Design review of the part shown in the three views and the two pictorial views. Dimensions are in mm from the part's minimum x, y and z. A direction names the side the tool comes from. Give positions to 0.01 mm unless a question says otherwise; leave off trailing zeros. Order: outer loops, then holes, each group sorted by start corner. A loop starts at its lowest first (then second) coordinate and runs counter-clockwise, first axis right, second up. Notation, with made-up numbers: (17.5, 66.5) -> (42.5, 66.5) arc R21 ccw to (42.5, 85.5) -> close; hole circle Ø5 at (51.5, 65.5). An arc over 180 degrees is marked (long way). Use one line per item in the form item = value.
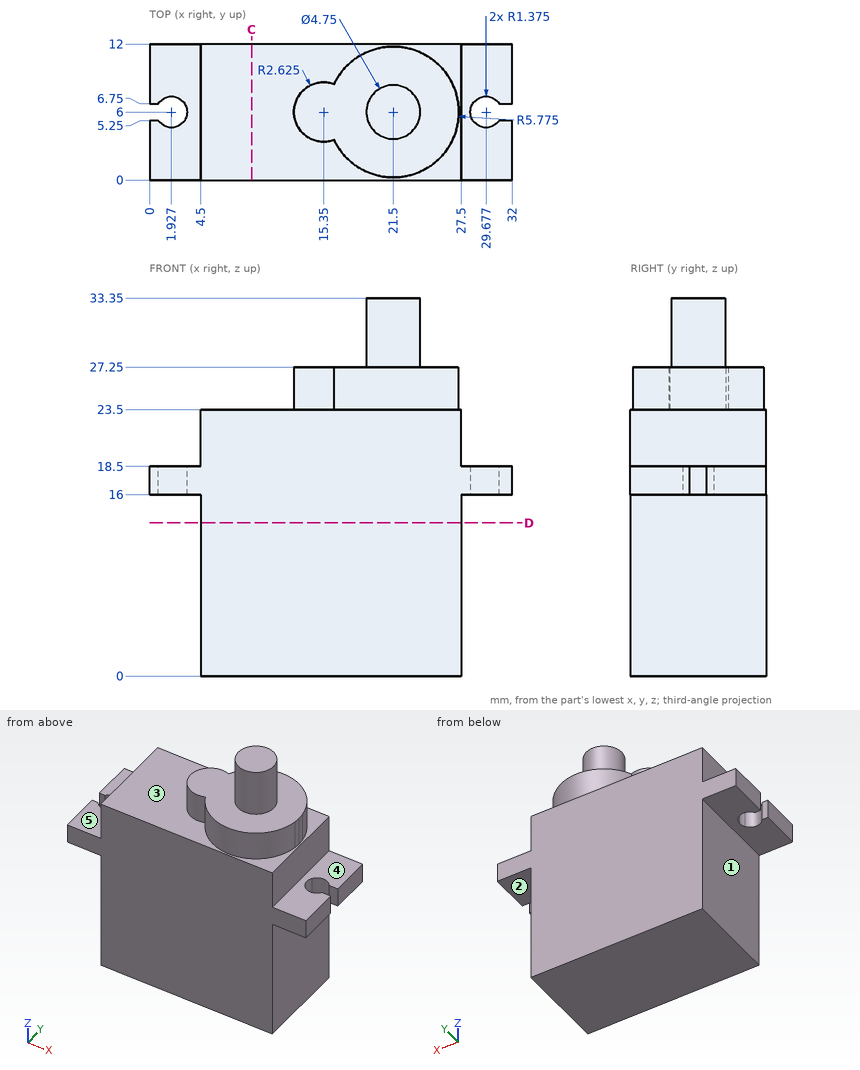
1. For pin 1 Ø3.5 at (x, y) = (30, 3.5) entering from -Z; pin 2 Ø1.5 at (y, z) = (4.5, 8) entering from +X; pin 3 Ø6 at (y, z) = (4.5, 4.5) entering from -X, all flat-tipped, find the tip position at first contact; note any pin that passes through.
Values:
pin_1 = 16
pin_2 = 27.5
pin_3 = 4.5
2. Add section C-C on x = 9. Give the boundary of the cut face in (y, z).
Values:
outline = (0, 0) -> (12, 0) -> (12, 23.5) -> (0, 23.5) -> close
3. Add section D-D on z = 13.5. Give the boundary of the cut face in (x, y), then the cut area to 3 significant figures.
Values:
outline = (4.5, 0) -> (27.5, 0) -> (27.5, 12) -> (4.5, 12) -> close
area = 276 mm^2
4. For L1, parallel to Z at x = 6, y = 1; L2, parallel to Z at x = 28, y = 8.5; L3, parallel to X at y = 9.5, z = 14, list the stretches that pass through material, from the lowest coordinate up.
Values:
L1 = 0 to 23.5
L2 = 16 to 18.5
L3 = 4.5 to 27.5
5. Tool access review of the marked faces 1, 2, 3, 4 and 5: name each direction out of +Z, -Z, +X, -X, +Y, -Y from which nothing blocks a thin tool from reaching the whole face with its end or side.
Values:
face_1 = -Z, -X, +Y, -Y
face_2 = -Z, +X, +Y, -Y
face_3 = +Z
face_4 = +Z, +X, +Y, -Y
face_5 = +Z, -X, +Y, -Y
